from build123d import *

# Parameters (mm, degrees)
SKETCH1_W           = 18.3
SKETCH1_H           = 6
BOSS_EXTRUDE1_DEPTH = 9
SKETCH2_W           = 15.6
SKETCH2_H           = 6.2
BOSS_EXTRUDE2_DEPTH = 49
SKETCH3_W           = 15.6
SKETCH3_H           = 8.5
BOSS_EXTRUDE3_DEPTH = 20.7
FILLET3_R           = 3
SKETCH4_W           = 31
SKETCH4_H           = 8
SKETCH4_H_2         = 6
BOSS_EXTRUDE4_DEPTH = 45
CUT_EXTRUDE1_DEPTH  = 58
SKETCH6_3_R         = 11.25
CUT_EXTRUDE2_DEPTH  = 6
CUT_EXTRUDE3_DEPTH  = 4.3
CUT_EXTRUDE4_DEPTH  = 2.2
SKETCH9_3_R         = 4.65
CUT_EXTRUDE5_DEPTH  = 8
SKETCH10_R          = 1.75
CUT_EXTRUDE6_DEPTH  = 18


with BuildPart() as part:
    # Sketch1 → Boss-Extrude1 (new body)
    with BuildSketch(Plane.XY):
        Polygon((15.5, -28.5), (-15.5, -28.5), (-15.5, -10.3), (-5.8, -10.3), (-5.8, 10.3), (-15.5, 10.3), (-15.5, 28.5), (15.5, 28.5), align=None)
        with Locations((0.65, -19.5)):
            Rectangle(SKETCH1_W, SKETCH1_H, mode=Mode.SUBTRACT)
    extrude(amount=BOSS_EXTRUDE1_DEPTH)

    # Sketch2 → Boss-Extrude2 (add)
    with BuildSketch(Plane.XY.offset(9)):
        with Locations((2, -13.4)):
            Rectangle(SKETCH2_W, SKETCH2_H)
        with Locations((2, 13.4)):
            Rectangle(SKETCH2_W, SKETCH2_H)
    extrude(amount=BOSS_EXTRUDE2_DEPTH)

    # Sketch3 → Boss-Extrude3 (add)
    with BuildSketch(Plane.XZ.offset(-10.3)):
        with Locations((2, 53.75)):
            Rectangle(SKETCH3_W, SKETCH3_H)
    extrude(amount=BOSS_EXTRUDE3_DEPTH)

    # Fillet3
    fillet3_edges = [part.edges().sort_by_distance(p)[0] for p in [
        (2, -16.5, 58),
    ]]
    fillet(fillet3_edges, radius=FILLET3_R)

    # Sketch4 → Boss-Extrude4 (add)
    with BuildSketch(Plane(origin=(0, 0, 0), x_dir=(-1, 0, 0), z_dir=(0, 0, -1))):
        with Locations((0, 24.5)):
            Rectangle(SKETCH4_W, SKETCH4_H)
        with Locations((0, -25.5)):
            Rectangle(SKETCH4_W, SKETCH4_H_2)
    extrude(amount=BOSS_EXTRUDE4_DEPTH)

    # Sketch6 → Cut-Extrude1 (cut, through all)
    with BuildSketch(Plane.XZ.offset(28.5)):
        with BuildLine():
            ThreePointArc((15.5, -29.5), (10.960155101, -40.460155116), (-2.1e-08, -45))
            Line((-2.1e-08, -45), (15.5, -45))
            Line((15.5, -45), (15.5, -29.5))
        make_face()
        with BuildLine():
            ThreePointArc((-2.1e-08, -45), (-10.960155116, -40.460155101), (-15.5, -29.5))
            Line((-15.5, -29.5), (-15.5, -45))
            Line((-15.5, -45), (-2.1e-08, -45))
        make_face()
    extrude(amount=-CUT_EXTRUDE1_DEPTH, mode=Mode.SUBTRACT)

    # Sketch6<3> → Cut-Extrude2 (cut)
    with BuildSketch(Plane.XZ.offset(28.5)):
        with Locations((0, -29.5)):
            Circle(SKETCH6_3_R)
    extrude(amount=-CUT_EXTRUDE2_DEPTH, mode=Mode.SUBTRACT)

    # Sketch7 → Cut-Extrude3 (cut)
    with BuildSketch(Plane(origin=(0, 28.5, 0), x_dir=(1, 0, 0), z_dir=(0, 1, 0))):
        with BuildLine():
            Line((-17.1, 31.65), (-4.313351365, 33.813351365))
            Line((-4.313351365, 33.813351365), (-2.15, 46.6))
            ThreePointArc((-2.15, 46.6), (0, 48.75), (2.15, 46.6))
            Line((2.15, 46.6), (4.313351365, 33.813351365))
            Line((4.313351365, 33.813351365), (17.1, 31.65))
            ThreePointArc((17.1, 31.65), (19.25, 29.5), (17.1, 27.35))
            Line((17.1, 27.35), (4.313351365, 25.186648635))
            Line((4.313351365, 25.186648635), (2.15, 12.4))
            ThreePointArc((2.15, 12.4), (0, 10.25), (-2.15, 12.4))
            Line((-2.15, 12.4), (-4.313351365, 25.186648635))
            Line((-4.313351365, 25.186648635), (-17.1, 27.35))
            ThreePointArc((-17.1, 27.35), (-19.25, 29.5), (-17.1, 31.65))
        make_face()
    extrude(amount=-CUT_EXTRUDE3_DEPTH, mode=Mode.SUBTRACT)

    # Sketch9 → Cut-Extrude4 (cut)
    with BuildSketch(Plane.XZ.offset(-20.5)):
        with BuildLine():
            ThreePointArc((3.25, -32.82565783), (0, -34.15), (-3.25, -32.82565783))
            Line((-3.25, -32.82565783), (-3.25, -44.655444566))
            ThreePointArc((-3.25, -44.655444566), (0, -45), (3.25, -44.655444566))
            Line((3.25, -44.655444566), (3.25, -32.82565783))
        make_face()
    extrude(amount=-CUT_EXTRUDE4_DEPTH, mode=Mode.SUBTRACT)

    # Sketch9<3> → Cut-Extrude5 (cut)
    with BuildSketch(Plane.XZ.offset(-20.5)):
        with Locations((0, -29.5)):
            Circle(SKETCH9_3_R)
    extrude(amount=-CUT_EXTRUDE5_DEPTH, mode=Mode.SUBTRACT)

    # Sketch10 → Cut-Extrude6 (cut)
    with BuildSketch(Plane.ZY.offset(5.8)):
        with Locations((4.5, 5)):
            Circle(SKETCH10_R)
        with Locations((4.5, -5)):
            Circle(SKETCH10_R)
        with Locations((53.75, 5)):
            Circle(SKETCH10_R)
        with Locations((53.75, -5)):
            Circle(SKETCH10_R)
    extrude(amount=-CUT_EXTRUDE6_DEPTH, mode=Mode.SUBTRACT)


solid = part.part
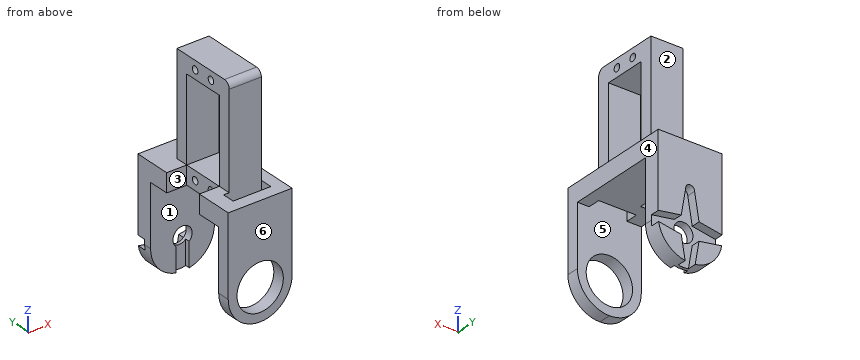
Could you check a few things on this model? Use its own coordinates, in mm. Face numbers are marked on the shaded views. A direction names the side the tool comes from. Coordinates: 2 decimals unless noted, no trailing zeros. Order: outer loops, then holes, each group sorted by start corner. A loop starts at its lowest first (then second) coordinate and runs counter-clockwise, first axis right, second up. Notation, with made-up numbers: (12.25, 68) - (16.25, 68) arc R20 cw to (16.25, 81) - close; hole circle Ø8 at (12, -22). An arc over 180 degrees is marked (long way). Answer in a Markdown table with one row per item. Add a question column.
(1) I need wall thicknesses on L1, parallel to Y at x = 0.75, z = 53.75; L2, parallel to Y at x = 2.75, z = 4.5; L3, parallel to Y at x = 6.5, z = -41. Which ranges of each line are inside material? Lowest first, please.
(2) If we mould it in two halves opening along X, with no side actions, what happens to the marked faces 4, 5 and 6? For each: released by +X, released by -X, zero draft, split by the parting line, or undercut.
(3) If we section it at D-D, the plane x = 1: State how many separate pieces and enclosed holes the cut face has, then the cut area to 3 significant figures.
(4) If we section it at B-B, the plane z = 26: Please give me the cut outline in (x, y), then the cut area to 3 significant figures.
(5) Will these pins go through, and if not, where does the flat tip stop? pin 1 (1 mm diameter, centred on y = 5, z = 5, fed in from -X); pin 2 (8 mm diameter, centred on x = 6, y = 14, fed in from -Z); pin 3 (2.5 mm diameter, centred on y = -2, z = 5.5, fed in from -X).
(6) If we section it at C-C, the plane z = 4.5: Please give me the cut outline in (x, y), then the cut area to 3 significant figures.
(7) If we section it at A-A, the plane y = 5: Please give me the cut outline in (x, z), then the cut area to 3 significant figures.
(8) On a 3-axis mill with a long thin cutter (end or side, diameter ignored), from which of +Z, -Z, +X, -X, +Y, -Y can I reach the whole of each face in a straight line? I mean the marked faces 1, 2 and 3. Say none if no direction works.
Results are:
| question | item | result |
|---|---|---|
| 1 | L1 | y = -16.5 to -6.75, -3.25 to 3.25, 6.75 to 16.5 |
| 1 | L2 | y = -28.5 to -22.5, -16.5 to -6.75, -3.25 to 3.25, 6.75 to 28.5 |
| 1 | L3 | y = -28.5 to -22.5, 20.5 to 28.5 |
| 2 | face 4 | released by +X |
| 2 | face 5 | undercut |
| 2 | face 6 | zero draft |
| 3 | separate pieces | 4 |
| 3 | enclosed holes | 5 |
| 3 | area | 1,490 mm2 |
| 4 | outline | (-5.8, -16.5) - (9.8, -16.5) - (9.8, -10.3) - (-5.8, -10.3) - close; (-5.8, 10.3) - (9.8, 10.3) - (9.8, 16.5) - (-5.8, 16.5) - close |
| 4 | area | 193 mm2 |
| 5 | pin 1 | stops at x = 12.2 |
| 5 | pin 2 | stops at z = 0 |
| 5 | pin 3 | stops at x = -5.8 |
| 6 | outline | (-15.5, -28.5) - (15.5, -28.5) - (15.5, 28.5) - (-15.5, 28.5) - (-15.5, 10.3) - (-5.8, 10.3) - (-5.8, 6.75) - (12.2, 6.75) - (12.2, 3.25) - (-5.8, 3.25) - (-5.8, -3.25) - (12.2, -3.25) - (12.2, -6.75) - (-5.8, -6.75) - (-5.8, -10.3) - (-15.5, -10.3) - close; hole (-8.5, -22.5) - (9.8, -22.5) - (9.8, -16.5) - (-8.5, -16.5) - close |
| 6 | area | 1,330 mm2 |
| 7 | outline | (-5.8, 0) - (15.5, 0) - (15.5, 9) - (-5.8, 9) - (-5.8, 6.25) - (12.2, 6.25) - (12.2, 2.75) - (-5.8, 2.75) - close; (-5.8, 49.5) - (9.8, 49.5) - (9.8, 52) - (-5.8, 52) - close; (-5.8, 55.5) - (9.8, 55.5) - (9.8, 58) - (-5.8, 58) - close |
| 7 | area | 207 mm2 |
| 8 | face 1 | -Z, +X, -X |
| 8 | face 2 | +Z, +X, -X, +Y |
| 8 | face 3 | +Z, -Z, -X |
